CAD build for the part. Positions are in the model's coordinates, mm. Give positions to 0.01 mm unless a question says otherwise; leave off trailing zeros. Loops run counter-clockwise (first coordinate to the right, second up) from the corner with the lowest first, then second, coordinate; pieces in that order, holes last. Notation, with made-up numbers: (42.5, 30) -> (78.5, 30) arc R16 cw to (78.5, 57) -> close; hole circle Ø3 at (-5, -14.5). An arc over 180 degrees is marked (long way). Write each question's results on one line, items separated by ' | '. Start each with the question number.
```python
from build123d import *

# Parameters (mm, degrees)
ESQUISSE1_W                  = 475
ESQUISSE1_H                  = 540
BOSS_EXTRU_1_DEPTH           = 8
ENL_V_MAT_EXTRU_1_DEPTH      = 720.228058407
ENL_V_MAT_EXTRU_1_DEPTH_BACK = 720.228058407
ESQUISSE2_R                  = 3.5
ENL_V_MAT_EXTRU_2_DEPTH      = 720.228058407
ENL_V_MAT_EXTRU_2_DEPTH_BACK = 720.228058407
ESQUISSE3_W                  = 120
ESQUISSE3_H                  = 45


with BuildPart() as part:
    # Esquisse1 → Boss.-Extru.1 (new body)
    with BuildSketch(Plane.XY):
        with Locations((237.5, 270)):
            Rectangle(ESQUISSE1_W, ESQUISSE1_H)
    extrude(amount=BOSS_EXTRU_1_DEPTH)

    # Esquisse2 → Enlèv. mat.-Extru.1 (cut, two sides: drawn at the far end of the back side and taken through both)
    with BuildSketch(Plane.XY.offset(8).offset(-ENL_V_MAT_EXTRU_1_DEPTH_BACK)):
        with Locations((160, 520)):
            Circle(ESQUISSE2_R)
        with Locations((40, 520)):
            Circle(ESQUISSE2_R)
        with Locations(Location((400, 520, 0), (0, 0, 180))):
            Circle(ESQUISSE2_R)
        with Locations(Location((280, 520, 0), (0, 0, 180))):
            Circle(ESQUISSE2_R)
        with Locations((280, 20)):
            Circle(ESQUISSE2_R)
        with Locations((400, 20)):
            Circle(ESQUISSE2_R)
        with Locations(Location((40, 20, 0), (0, 0, 180))):
            Circle(ESQUISSE2_R)
        with Locations(Location((160, 20, 0), (0, 0, 180))):
            Circle(ESQUISSE2_R)
    extrude(amount=ENL_V_MAT_EXTRU_1_DEPTH + ENL_V_MAT_EXTRU_1_DEPTH_BACK, mode=Mode.SUBTRACT)

    # Esquisse3 → Enlèv. mat.-Extru.2 (cut, two sides: drawn at the far end of the back side and taken through both)
    with BuildSketch(Plane.XY.offset(8).offset(-ENL_V_MAT_EXTRU_2_DEPTH_BACK)):
        with Locations((415, 517.5)):
            Rectangle(ESQUISSE3_W, ESQUISSE3_H)
        with Locations((415, 22.5)):
            Rectangle(ESQUISSE3_W, ESQUISSE3_H)
    extrude(amount=ENL_V_MAT_EXTRU_2_DEPTH + ENL_V_MAT_EXTRU_2_DEPTH_BACK, mode=Mode.SUBTRACT)


solid = part.part
```
Q1. Saw through at A-A, the plane z = 2. List the corners of the cut face in (x, y).
Q2. Saw through at B-B, the plane x = 411. List the corners of the cut face in (y, z), then the cut area to 3 significant figures.
Q3. Drop a flat-ended pin along its axis: pin 1 (4 mm diameter, centred on y = 15.5, z = 4.5, fed in from +X). Give the stop position or say it passes through.
Q4. Wall check: L1, parallel to Y at x = 40, z = 5; L2, parallel to X at y = 520, z = 1.5; L3, parallel to Y at x = 449.5, z = 6.75. Give the ranges that are in metal, low to high.
Q5. Saw through at C-C, the plane y = 33.5. List the corners of the cut face in (x, z), then the cut area to 3 significant figures.
Answer block:
1) outline: (0, 0) -> (355, 0) -> (355, 45) -> (475, 45) -> (475, 495) -> (355, 495) -> (355, 540) -> (0, 540) -> close; hole circle Ø7 at (40, 20); hole circle Ø7 at (40, 520); hole circle Ø7 at (160, 20); hole circle Ø7 at (160, 520); hole circle Ø7 at (280, 20); hole circle Ø7 at (280, 520)
2) outline: (45, 0) -> (495, 0) -> (495, 8) -> (45, 8) -> close | area: 3,600 mm2
3) pin 1: stops at x = 355
4) L1: y = 0 to 16.5, 23.5 to 516.5, 523.5 to 540 | L2: x = 0 to 36.5, 43.5 to 156.5, 163.5 to 276.5, 283.5 to 355 | L3: y = 45 to 495
5) outline: (0, 0) -> (355, 0) -> (355, 8) -> (0, 8) -> close | area: 2,840 mm2
